Read the model definition and answer for the solid it produces. Units are mm, in the model's axes. A direction names the side the tool comes from. Coordinates: 2 decimals unless noted, no trailing zeros. Order: outer loops, then holes, each group sorted by start corner. A loop starts at its lowest first (then second) coordinate and runs counter-clockwise, first axis right, second up. Notation, with made-up numbers: M -17.5,55 L 6.5,55 A24 ccw 6.5,78 Z; hole C 63.25,8 d3. An arc over 180 degrees is marked long. Use a Markdown table: item, result. Add a question column.
1) Find section C-C on y = 3. Write down the section's boundary in (x, z).
2) Each of these flat-tipped pins is pushed along its axis until it touches: pin 1 Ø3 at (x, z) = (18.5, 3.5) entering from -Y; pin 2 Ø2 at (y, z) = (11.5, 5) entering from +X. Where does it stop, or does it pass through?
3) Find section D-D on z = 1.5. Write down the section's boundary in (x, y) (3 decimals), plus the area to 3 significant figures.
4) For faces 1 (the face through (40, 8.014, 5)), 2 (the face through (41, 0, 3)), determine the directions among +Z, -Z, +X, -X, +Y, -Y from which every point of the face is accessible in a straight line to the end or side of a thin tool.
5) Find the intervals of material crossed by probe 1 along Y at (x, z) = (41.5, 5.75) (1 decimal); probe 2 along Z at (x, y) = (48.5, 7.75); probe 3 along X at (y, z) = (4, 5.5), in increasing order. Write a range as [from, to].
from build123d import *

# Parameters (mm, degrees)
BOSS_EXTRUDE1_DEPTH     = 28.575
SKETCH2_W               = 2.9972
SKETCH2_H               = 3.2512
CUT_EXTRUDE1_DEPTH      = 82.0006
CUT_EXTRUDE1_DEPTH_BACK = 1


with BuildPart() as part:
    # Sketch1 → Boss-Extrude1 (new body)
    with BuildSketch(Plane(origin=(0, 0, 0), x_dir=(1, 0, 0), z_dir=(0, 1, 0))):
        Polygon((0, 0), (81.0006, 0), (74.6506, -6.35), (6.35, -6.35), align=None)
    extrude(amount=BOSS_EXTRUDE1_DEPTH)

    # Sketch2 → Cut-Extrude1 (cut, two sides)
    with BuildSketch(Plane(origin=(0, 0, 0), x_dir=(0, 0, -1), z_dir=(1, 0, 0))) as cut_extrude1_sk:
        with Locations((-4.8514, 6.3881)):
            Rectangle(SKETCH2_W, SKETCH2_H)
    extrude(amount=CUT_EXTRUDE1_DEPTH, mode=Mode.SUBTRACT)
    extrude(cut_extrude1_sk.sketch, amount=-CUT_EXTRUDE1_DEPTH_BACK, mode=Mode.SUBTRACT)


solid = part.part
Check result:
| question | item | result |
|---|---|---|
| 1 | outline | M 0,0 L 81,0 L 74.65,6.35 L 6.35,6.35 Z |
| 2 | pin 1 | stops at y = 0 |
| 2 | pin 2 | stops at x = 77 |
| 3 | outline | M 1.5,0 L 79.501,0 L 79.501,28.575 L 1.5,28.575 Z |
| 3 | area | 2,230 mm2 |
| 4 | face 1 | +Z, +X, -X |
| 4 | face 2 | +Z, -Z, +X, -X, -Y |
| 5 | probe 1 | y = [0, 4.8], [8, 28.6] |
| 5 | probe 2 | z = [0, 3.35] |
| 5 | probe 3 | x = [5.5, 75.5] |
